from build123d import *

# Parameters (mm, degrees)
BOSS_EXTRUDE1_DEPTH = 12


with BuildPart() as part:
    # Sketch1 → Boss-Extrude1 (new body)
    with BuildSketch(Plane(origin=(0, 0, 0), x_dir=(1, 0, 0), z_dir=(0, 1, 0))):
        with BuildLine():
            Line((7.550302589, -2.572347999), (6.903132735, -4.464746261))
            ThreePointArc((6.903132735, -4.464746261), (19.502585792, 8.507647316), (1.480319122, 10))
            Line((1.480319122, 10), (0, 10))
            Line((0, 10), (0, 0))
            Line((0, 0), (4, 0))
            Line((4, 0), (4, 10))
            Line((4, 10), (3.89619073, 10))
            ThreePointArc((3.89619073, 10), (17.821084722, 7.230023098), (7.550302589, -2.572347999))
        make_face()
    extrude(amount=BOSS_EXTRUDE1_DEPTH)


solid = part.part
Can you work these out from the model? Positions are in its coordinate system, mm. A direction names the side the tool comes from. Give positions to 0.01 mm unless a question says otherwise; leave off trailing zeros. Loops run counter-clockwise (first coordinate to the right, second up) from the corner with the lowest first, then second, coordinate; pieces in that order, holes last. Notation, with made-up numbers: (40, 20.5) - (48, 20.5) arc R21 cw to (48, 37.5) - close; hole circle Ø9 at (-18.75, 77). An arc over 180 degrees is marked (long way). One line per item, written item: value.
(1) On a 3-axis mill with a long thin cutter (end or side, diameter ignored), from which of +Z, -Z, +X, -X, +Y, -Y can I reach the whole of each face in a straight line? I mean faces 4 (the face through (2, 6, 0)), 5 (the face through (7.23, 5.92, 3.51)), 6 (the face through (3, 12, -6)). Say none if no direction works.
Verdict:
face 4: +Z, -X, +Y, -Y
face 5: -X, +Y, -Y
face 6: +Z, -Z, +X, -X, +Y
(2) If we section it at D-D, the plane x = 3.25: List the corners of the cut face in (y, z) for me, plus the area to 3 significant figures.
Verdict:
outline: (0, -12.25) - (12, -12.25) - (12, 0) - (0, 0) - close
area: 147 mm^2
(3) If we section it at B-B, the plane x = 17.75: List the corners of the cut face in (y, z) for me, plus the area to 3 significant figures.
Verdict:
outline: (0, -11.48) - (12, -11.48) - (12, -7.46) - (0, -7.46) - close; (0, -2.53) - (12, -2.53) - (12, 1.49) - (0, 1.49) - close
area: 96.5 mm^2
(4) I'm going to push flat-ended pins straight in: pin 1 (1.5 mm diameter, centred on x = 5.5, z = 1, fed in from +Y); pin 2 (1.5 mm diameter, centred on x = 8, y = 4.5, fed in from +Z); pin 3 (1.2 mm diameter, centred on x = 2.5, y = 7, fed in from +Z); pin 4 (0.7 mm diameter, centred on x = 1, y = 3.5, fed in from -Z). Where does each tip first touch, or does it pass through?
Verdict:
pin 1: through
pin 2: z = 4.91
pin 3: z = 0
pin 4: z = -10
(5) I need wall thicknesses on line 1 along Z through (x, y) = (10.25, 1.5); line 2 along X through (y, z) = (1, -1.25); line 3 along X through (y, z) = (1.25, -3.5). Which ranges of each line are inside material? Lowest first, please.
Verdict:
line 1: -15 to -13, 3 to 5
line 2: 0 to 4, 17.21 to 19.41
line 3: 0 to 4, 18 to 20.03
(6) If we section it at C-C, the plane y = 7.25: List the corners of the cut face in (x, z) for me, plus the area to 3 significant figures.
Verdict:
outline: (0, -10) - (1.48, -10) arc R10 ccw (long way) to (6.9, 4.46) - (7.55, 2.57) arc R8 cw (long way) to (3.9, -10) - (4, -10) - (4, 0) - (0, 0) - close
area: 120 mm^2
(7) If we section it at A-A, the plane z = -5: List the corners of the cut face in (x, y) for me, plus the area to 3 significant figures.
Verdict:
outline: (0, 0) - (4, 0) - (4, 12) - (0, 12) - close; (18.14, 0) - (20.14, 0) - (20.14, 12) - (18.14, 12) - close
area: 72.0 mm^2
(8) If we mould it in two halves opening along X, with no side actions, what happens to faces 1 (the face through (1, 6, -10)), 2 (the face through (19.61, 5.92, -8.21)), 3 (the face through (4, 6, -5))? For each: released by +X, released by -X, zero draft, split by the parting line, or undercut.
Verdict:
face 1: zero draft
face 2: split by the parting line
face 3: undercut
